Model file for the job. Use its own axes, mm. Coordinates: 2 decimals unless noted, no trailing zeros. Loops run counter-clockwise (first coordinate to the right, second up) from the corner with the lowest first, then second, coordinate; pieces in that order, holes last. Notation, with made-up numbers: (-12, 70.25) -> (47, 70.25) arc R32 cw to (47, 102.25) -> close; hole circle Ø7 at (39, -32.5). An arc over 180 degrees is marked (long way). Use one line per item in the form item = value.
```python
from build123d import *

# Parameters (mm, degrees)
F1_DEPTH = 2
F2_R     = 2.5
F3_DEPTH = 25
F4_SIZE  = 0.5
F5_SIZE  = 0.5
F6_R     = 0.4
F8_DEPTH = 0.4


with BuildPart() as f1:
    # F0 (on Top) → F1 (new body)
    with BuildSketch(Plane.XY):
        Polygon((1.5653009757, -10), (1.5653009757, 0), (-86.3636312124, 0), (-98.4346990243, -5), (-86.3636312124, -10), align=None)
    extrude(amount=F1_DEPTH)

    # F2 (on face) → F3 (cut)
    with BuildSketch(Plane.XY.offset(2)):
        with Locations((-68.4346990243, -5)):
            Circle(F2_R)
    extrude(amount=-F3_DEPTH, mode=Mode.SUBTRACT)

    # F4
    f4_edges = [f1.edges().sort_by_distance(p)[0] for p in [
        (-70.934699, -5, 2),
        (-70.934699, -5, 0),
    ]]
    chamfer(f4_edges, length=F4_SIZE)

    # F5
    f5_edges = [f1.edges().sort_by_distance(p)[0] for p in [
        (1.565301, -5, 2),
        (1.565301, -5, 0),
    ]]
    chamfer(f5_edges, length=F5_SIZE)

    # F6
    f6_edges = [f1.edges().sort_by_distance(p)[0] for p in [
        (-98.434699, -5, 1),
    ]]
    fillet(f6_edges, radius=F6_R)

    # F7 (on face) → F8 (join)
    with BuildSketch(Plane.XY.offset(2)):
        with BuildLine():
            ThreePointArc((-97.5425220254, -5.369551813), (-97.4674847812, -5.3923141122), (-97.3894486524, -5.4))
            Line((-97.3894486524, -5.4), (-92.3894486524, -5.4))
            ThreePointArc((-92.3894486524, -5.4), (-91.9894486524, -5), (-92.3894486524, -4.6))
            Line((-92.3894486524, -4.6), (-97.3894486524, -4.6))
            ThreePointArc((-97.3894486524, -4.6), (-97.4674847812, -4.6076858878), (-97.5425220254, -4.630448187))
            ThreePointArc((-97.5425220254, -4.630448187), (-97.7894486524, -5), (-97.5425220254, -5.369551813))
        make_face()
    extrude(amount=F8_DEPTH)


solid = f1.part
```
Q1. Pin check, flat tips, straight feed: pin 1 Ø1.5 at (x, y) = (-46.5, -8.5) entering from -Z; pin 2 Ø3 at (x, y) = (-41.5, -7.5) entering from +Z; pin 3 Ø4.5 at (x, y) = (-68.43, -5) entering from +Z. Stop position of each tip, or through.
Result:
pin_1 = 0
pin_2 = 2
pin_3 = through
Q2. Mould opens along X. For faces 1 (the face through (-42, 0, 1)), 2 (the face through (-70.932, -4.89, 1.007)), 3 (the face through (-92.031, -7.652, 0.986)) say: released by +X, released by -X, zero draft, split by the parting line, or undercut.
Result:
face_1 = zero draft
face_2 = undercut
face_3 = released by -X
Q3. Wall check: line 1 along Z through (x, y) = (-75, -6.5); line 2 along X through (y, z) = (-7.25, 0.8); line 3 along X through (y, z) = (-2, 1.95). Give the ranges that are in metal, low to high.
Result:
line_1 = 0 to 2
line_2 = -93 to -69.52, -67.34 to 1.57
line_3 = -91.19 to 1.12
Q4. Band-saw the part on A-A, the plane x = -72.5. Write the cut outline in (y, z), and give its area (3 significant figures).
Result:
outline = (-10, 0) -> (0, 0) -> (0, 2) -> (-10, 2) -> close
area = 20.0 mm2
